```python
from build123d import *

# Parameters (mm, degrees)
SKETCH1_R           = 2.5
BOSS_EXTRUDE1_DEPTH = 30
FILLET1_R           = 5
SKETCH2_R           = 2.75
CUT_EXTRUDE1_DEPTH  = 124


with BuildPart() as part:
    # Sketch1 → Boss-Extrude1 (new body)
    with BuildSketch(Plane(origin=(0, 0, 0), x_dir=(1, 0, 0), z_dir=(0, 1, 0))):
        with BuildLine():
            Line((-5, 30), (-5, 10))
            ThreePointArc((-5, 10), (-3.535533906, 6.464466094), (0, 5))
            ThreePointArc((0, 5), (5, 0), (0, -5))
            ThreePointArc((0, -5), (-7.071067812, -2.071067812), (-10, 5))
            Line((-10, 5), (-10, 30))
            Line((-10, 30), (-5, 30))
        make_face()
        with Locations(Location((0, 0, 0), (0, 0, 270))):
            Circle(SKETCH1_R, mode=Mode.SUBTRACT)
    extrude(amount=BOSS_EXTRUDE1_DEPTH)

    # Fillet1
    fillet1_edges = [part.edges().sort_by_distance(p)[0] for p in [
        (-10, 15, -30),
    ]]
    fillet(fillet1_edges, radius=FILLET1_R - 0.0001)  # a hair under: the kernel refuses the full size

    # Sketch2 → Cut-Extrude1 (cut)
    with BuildSketch(Plane(origin=(5, -405, -405), x_dir=(0, 0, -1), z_dir=(1, 0, 0))):
        with Locations((-376.5, 410)):
            Circle(SKETCH2_R)
    extrude(amount=-CUT_EXTRUDE1_DEPTH, mode=Mode.SUBTRACT)


solid = part.part
```
Could you check a few things on this model? Use its own coordinates, in mm. A direction names the side the tool comes from. Give positions to 0.01 mm unless a question says otherwise; leave off trailing zeros. Loops run counter-clockwise (first coordinate to the right, second up) from the corner with the lowest first, then second, coordinate; pieces in that order, holes last. Notation, with made-up numbers: (-30, -38.75) - (26, -38.75) arc R26 ccw to (26, -8.75) - close; hole circle Ø11 at (55.25, 79). An arc over 180 degrees is marked (long way). Use one line per item in the form item = value.
1. I'm going to push flat-ended pins straight in: pin 1 Ø6 at (x, y) = (-2.5, 13) entering from +Z; pin 2 Ø8 at (x, y) = (0.5, 14) entering from -Z; pin 3 Ø6 at (y, z) = (12, -24) entering from +X; pin 4 Ø5 at (x, z) = (-2, -17) entering from -Y. Where does each tip first touch, or does it pass through?
Response values:
pin_1 = 5
pin_2 = -6.43
pin_3 = -5
pin_4 = through
2. I want a section at C-C (z = -28.5). Please give me the cut outline in (x, y).
Response values:
outline = (-8.57, 0) - (-5, 0) - (-5, 2.25) - (-8.57, 2.25) - close; (-8.57, 7.75) - (-5, 7.75) - (-5, 30) - (-8.57, 30) - close
3. I need wall thicknesses on probe 1 along Y at (x, z) = (-7.95, -28.5); probe 2 along X at (y, z) = (13, -24.5); probe 3 along Z at (x, y) = (1.5, 12). Which ranges of each line are inside material? Lowest first, please.
Response values:
probe_1 = 0 to 2.25, 7.75 to 30
probe_2 = -10 to -5
probe_3 = -4.77 to -2, 2 to 4.77
4. I want a section at D-D (z = -20). Please give me the cut outline in (x, y), and give its area (3 significant figures).
Response values:
outline = (-10, 0) - (-5, 0) - (-5, 30) - (-10, 30) - close
area = 150 mm²
5. I want a section at B-B (x = 0.5). Please give me the cut outline in (y, z).
Response values:
outline = (0, -4.97) - (30, -4.97) - (30, -2.45) - (0, -2.45) - close; (0, 2.45) - (30, 2.45) - (30, 4.97) - (0, 4.97) - close
6. Thinking about a two-plate mould opening in Z: for faces 1 (the face through (-10, 15, -15)), 2 (the face through (-6.99, 14.79, 2.15)), 3 (the face through (-2.44, 14.79, -0.54)), 4 (the face through (-6.89, 5.08, -25.75)), which applies, released by +Z, released by -Z, zero draft, split by the parting line, or undercut?
Response values:
face_1 = zero draft
face_2 = released by +Z
face_3 = undercut
face_4 = undercut
7. On a 3-axis mill with a long thin cutter (end or side, diameter ignored), from which of +Z, -Z, +X, -X, +Y, -Y can I reach the whole of each face in a straight line? I mean faces 5 (the face through (-5, 15, -20)), 6 (the face through (-6, 30, -9)). Say none if no direction works.
Response values:
face_5 = -Z, +X, +Y, -Y
face_6 = +Z, -Z, +X, -X, +Y
